Part model, mm, in its own coordinate system. A direction names the side the tool comes from. Coordinates: 2 decimals unless noted, no trailing zeros. Order: outer loops, then holes, each group sorted by start corner. A loop starts at its lowest first (then second) coordinate and runs counter-clockwise, first axis right, second up.
Autodesk Fusion 360 part; units mm, degrees
sketch "Sketch1" plane through (0, 0, 0) normal (0, 1, 0) x (1, 0, 0)
  circle A0 centre (0, 0) radius 10
  circle A1 centre (0, 0) radius 2.7
  line L0 (2.7, -1.8) -> (-2.7, -1.8)
  line L1 (-2.7, -1.8) -> (-2.7, 1.8)
  line L2 (-2.7, 1.8) -> (2.7, 1.8)
  line L3 (2.7, 1.8) -> (2.7, -1.8)
  line L4 (2.7, -1.8) -> (-2.7, 1.8) construction
  line L5 (-2.7, -1.8) -> (2.7, 1.8) construction
  dimension "d1" = 20
  dimension "d2" = 5.4
  dimension "d3" = 5.4
  dimension "d4" = 3.6
extrude "Extrude1" add sketch "Sketch1" along normal blind 4.4 contours A0 | A1 L0 L3 | A1 L2 L3 | A1 L2 | A1 L0 | A1 L1 L2 | A1 L0 L1
sketch "Sketch4" plane through (0, 0, 0) normal (0, 1, 0) x (1, 0, 0)
  arc A0 (2.0125, -1.8) -> (2.0125, 1.8) centre (0, 0) ccw
  line L0 (2.0125, 1.8) -> (-2.0125, 1.8)
  arc A1 (-2.0125, 1.8) -> (-2.0125, -1.8) centre (0, 0) ccw
  line L1 (-2.0125, -1.8) -> (2.0125, -1.8)
  circle A2 centre (0, 0) radius 10
Q1. Cut at D-D on z = 3.5. Write the cut outline in (x, y), and give its area (3 significant figures).
Results list:
outline: (-9.37, 0) - (9.37, 0) - (9.37, 4.4) - (-9.37, 4.4) - close
area: 82.4 mm2
Q2. Cut at C-C on y = 2. Write the cut outline in (x, z).
Results list:
outline: circle Ø20 at (0, 0); hole (-2.01, -1.8) - (2.01, -1.8) arc R2.7 ccw to (2.01, 1.8) - (-2.01, 1.8) arc R2.7 ccw to start
Q3. Cut at B-B on x = 0. Write the cut outline in (y, z).
Results list:
outline: (0, -10) - (4.4, -10) - (4.4, -1.8) - (0, -1.8) - close; (0, 1.8) - (4.4, 1.8) - (4.4, 10) - (0, 10) - close
Q4. Pin check, flat tip, straight feed: pin 1 Ø1 at (x, y) = (-3, 1) entering from -Z. Stop position of the tip, or through.
Results list:
pin 1: stops at z = -9.68
Q5. Mould opens along Z. For faces 1 (the face through (-2.7, 2.2, 0)), 2 (the face through (-2.17, 2.17, -9.76)), 3 (the face through (0, 4.4, 2)) say: pulls with the +Z half, pulls with the -Z half, needs draft (parallel to the pull), parting line crosses it, or undercut.
Results list:
face 1: undercut
face 2: parting line crosses it
face 3: needs draft
Q6. Wall check: line 1 along X through (y, z) = (3.3, 0.75); line 2 along X through (y, z) = (2.35, -9). Give the ranges that are in metal, low to high.
Results list:
line 1: x = -9.97 to -2.59, 2.59 to 9.97
line 2: x = -4.36 to 4.36
Q7. Cut at A-A on z = 0. Write the cut outline in (x, y).
Results list:
outline: (-10, 0) - (-2.7, 0) - (-2.7, 4.4) - (-10, 4.4) - close; (2.7, 0) - (10, 0) - (10, 4.4) - (2.7, 4.4) - close
Q8. Which spindle directions (+Z, -Z, +X, -X, +Y, -Y) get a long thin tool onto all of the face, cutting with end or side? Do faces 4 (the face through (0, 0, 2)), 5 (the face through (0, 2, 1.8)). Say none if no direction does.
Results list:
face 4: +Z, -Z, +X, -X, -Y
face 5: +Y, -Y
